Part model, mm, in its own coordinate system. A direction names the side the tool comes from. Round coordinates to 2 decimals unless told otherwise and drop trailing zeros. Loops run counter-clockwise (first coordinate to the right, second up) from the corner with the lowest first, then second, coordinate; pieces in that order, holes last. Notation, with made-up numbers: M 36,77.5 L 55,77.5 A15 ccw 55,84.5 Z; hole C 25.5,20.25 d1. An arc over 180 degrees is marked long. Put each result on its own line as item: value. Start each with the question number.
```python
from build123d import *

# Parameters (mm, degrees)
BOSS_EXTRUDE2_START  = 12.7
BOSS_EXTRUDE2_DEPTH  = 12.7
BOSS_EXTRUDE3_DEPTH  = 12.7
SKETCH8_R            = 0.9525
CUT_EXTRUDE1_DEPTH   = 157.544227843
SKETCH9_R            = 0.9525
CUT_EXTRUDE2_DEPTH   = 164.292861742
SKETCH12_R           = 2.5527
BOSS_EXTRUDE10_DEPTH = 3.175


with BuildPart() as part:
    # Sweep1: sweep along a path in Sketch4
    with BuildLine(Plane.XY) as sweep1_path:
        Line((0, 0), (0, -92.964))
        ThreePointArc((0, -92.964), (0.223184633, -93.502815367), (0.762, -93.726))
        Line((0.762, -93.726), (93.726, -93.726))
    # Sketch3 → Sweep1 (sweep)
    with BuildSketch(Plane(origin=(0, 0, 0), x_dir=(1, 0, 0), z_dir=(0, 1, 0))):
        with BuildLine():
            Line((0, 16.62500014), (-25.4, 16.62500014))
            Line((-25.4, 16.62500014), (-25.4, 10.27500014))
            Line((-25.4, 10.27500014), (-6.985, 10.27500014))
            ThreePointArc((-6.985, 10.27500014), (-6.535987194, 10.089012946), (-6.35, 9.64000014))
            Line((-6.35, 9.64000014), (-6.35, -14.48999986))
            ThreePointArc((-6.35, -14.48999986), (-6.535987194, -14.939012666), (-6.985, -15.12499986))
            Line((-6.985, -15.12499986), (-25.4, -15.12499986))
            Line((-25.4, -15.12499986), (-25.4, -21.47499986))
            Line((-25.4, -21.47499986), (0, -21.47499986))
            Line((0, -21.47499986), (0, 16.62500014))
        make_face()
    sweep(path=sweep1_path.line)

    # Sketch6 → Boss-Extrude2 (add)
    with BuildSketch(Plane(origin=(93.726, 0, 0), x_dir=(0, 0, -1), z_dir=(1, 0, 0)).offset(BOSS_EXTRUDE2_START)):
        with BuildLine():
            Line((-18.04599986, -97.155), (13.19600014, -97.155))
            Line((13.19600014, -97.155), (13.19600014, -119.126))
            Line((13.19600014, -119.126), (10.27500014, -119.126))
            Line((10.27500014, -119.126), (10.27500014, -100.711))
            ThreePointArc((10.27500014, -100.711), (10.089012946, -100.261987194), (9.64000014, -100.076))
            Line((9.64000014, -100.076), (-14.48999986, -100.076))
            ThreePointArc((-14.48999986, -100.076), (-14.939012666, -100.261987194), (-15.12499986, -100.711))
            Line((-15.12499986, -100.711), (-15.12499986, -119.126))
            Line((-15.12499986, -119.126), (-18.04599986, -119.126))
            Line((-18.04599986, -119.126), (-18.04599986, -97.155))
        make_face()
    extrude(amount=-BOSS_EXTRUDE2_DEPTH)

    # Sketch7 → Boss-Extrude3 (add)
    with BuildSketch(Plane(origin=(0, 0, 0), x_dir=(1, 0, 0), z_dir=(0, 1, 0))):
        Polygon((-25.4, 13.45000014), (-25.4, 16.62500014), (0, 16.62500014), (0, -21.47499986), (-25.4, -21.47499986), (-25.4, -18.29999986), (-3.175, -18.29999986), (-3.175, 13.45000014), align=None)
    extrude(amount=BOSS_EXTRUDE3_DEPTH)

    # Sketch8 → Cut-Extrude1 (cut, through all)
    with BuildSketch(Plane.XZ.offset(100.076)):
        with Locations(Location((100.076, 8.13999986, 0), (0, 0, 270))):
            Circle(SKETCH8_R)
        with Locations(Location((100.076, -3.29000014, 0), (0, 0, 270))):
            Circle(SKETCH8_R)
    extrude(amount=-CUT_EXTRUDE1_DEPTH, mode=Mode.SUBTRACT)

    # Sketch9 → Cut-Extrude2 (cut, through all)
    with BuildSketch(Plane.ZY.offset(3.175)):
        with Locations((-3.29000014, 6.35)):
            Circle(SKETCH9_R)
        with Locations((8.13999986, 6.35)):
            Circle(SKETCH9_R)
    extrude(amount=-CUT_EXTRUDE2_DEPTH, mode=Mode.SUBTRACT)

    # Sketch12 → Boss-Extrude10 (add, symmetric)
    with BuildSketch(Plane.XY.offset(7.62)):
        with BuildLine():
            Line((0.762, -93.726), (25.622204075, -93.726))
            ThreePointArc((25.622204075, -93.726), (18.183696875, -75.542303125), (0, -68.103795925))
            Line((0, -68.103795925), (0, -92.964))
            ThreePointArc((0, -92.964), (0.223184633, -93.502815367), (0.762, -93.726))
        make_face()
        with Locations((11.43, -82.296)):
            Circle(SKETCH12_R, mode=Mode.SUBTRACT)
    extrude(amount=BOSS_EXTRUDE10_DEPTH, both=True)

    # Sketch14 → CSK for _6 Flat Head Machine Screw _100 (revolve, cut)
    with BuildSketch(Plane(origin=(100.076, -100.076, -3.29000014), x_dir=(0, 0, -1), z_dir=(1, 0, 0))):
        Polygon((0, 0), (0, 2.410824014), (1.89865, 1.27), (1.89865, 1.380025208), (3.5433, 0), align=None)
    revolve(axis=Axis((100.076, -106.426, -3.29000014), (0, 1, 0)), mode=Mode.SUBTRACT)

    # Sketch16 → CSK for _6 Flat Head Machine Screw _ 2 (revolve, cut)
    with BuildSketch(Plane(origin=(100.076, -100.076, 8.13999986), x_dir=(0, 0, -1), z_dir=(1, 0, 0))):
        Polygon((0, 0), (0, 2.410824014), (1.89865, 1.27), (1.89865, 1.380025208), (3.5433, 0), align=None)
    revolve(axis=Axis((100.076, -106.426, 8.13999986), (0, 1, 0)), mode=Mode.SUBTRACT)


solid = part.part
```
1. Cut at A-A, the plane y = -49. Give the cut face in (x, z) (3 decimals), and give its area (3 significant figures).
2. Mould opens along X. For faces 1 (the flat face through (93.726, -97, 1)), 2 (the flat face through (-14, 6, 18.3)), 3 (the cylindrical face through (-17.9, -111.3, -13.4)), 4 (the cylindrical face through (11.098, -79.765, 7.576)) say: released by +X, released by -X, zero draft, split by the parting line, or undercut.
3. Which spindle directions (+Z, -Z, +X, -X, +Y, -Y) get a long thin tool onto all of the face, cutting with end or side? Do faces 5 (the flat face through (-14, 6, -13.45)), 6 (the flat face through (100, -108, -13.196)), 7 (the flat face through (10, -86, 10.795)). Say none if no direction does.
4. Cut at B-B, the plane x = 60. Give the cut face in (y, z) (3 decimals).
5. Cut at C-C, the plane x = 11.43. Give the cut face in (y, z) (3 decimals), and give its area (3 significant figures).
6. Wall check: L1, parallel to Z at x = 57.5, y = -108 (3 decimals); L2, parallel to Z at x = 96.5, y = -105 (3 decimals); L3, parallel to X at y = -97.55, z = -3.29. Give the ranges that are in metal, low to high.
7. Drop flat-ended pins along their axis: pin 1 (4 mm diameter, centred on y = -53, z = 12.5, fed in from +X); pin 2 (10 mm diameter, centred on x = 100.5, z = 5.5, fed in from +Y) (3 decimals); pin 3 (4 mm diameter, centred on y = -3, z = -0.5, fed in from -X). Give the stop position or say it passes through.
Results list:
1. outline: M -25.4,-16.625 L 0,-16.625 L 0,21.475 L -25.4,21.475 L -25.4,15.125 L -6.985,15.125 A0.635 cw -6.35,14.49 L -6.35,-9.64 A0.635 cw -6.985,-10.275 L -25.4,-10.275 Z
1. area: 484 mm^2
2. face 1: released by +X
2. face 2: zero draft
2. face 3: released by -X
2. face 4: undercut
3. face 5: -X, +Y
3. face 6: -Z, +X, +Y, -Y
3. face 7: +Z, +X, +Y
4. outline: M -119.126,-16.625 L -93.726,-16.625 L -93.726,21.475 L -119.126,21.475 L -119.126,15.125 L -100.711,15.125 A0.635 cw -100.076,14.49 L -100.076,-9.64 A0.635 cw -100.711,-10.275 L -119.126,-10.275 Z
5. outline: M -119.126,-16.625 L -93.726,-16.625 L -93.726,4.445 L -84.849,4.445 L -84.849,10.795 L -93.726,10.795 L -93.726,21.475 L -119.126,21.475 L -119.126,15.125 L -100.711,15.125 A0.635 cw -100.076,14.49 L -100.076,-9.64 A0.635 cw -100.711,-10.275 L -119.126,-10.275 Z; M -79.743,4.445 L -70.709,4.445 L -70.709,10.795 L -79.743,10.795 Z
5. area: 598 mm^2
6. L1: z = -16.625 to -10.275, 15.125 to 21.475
6. L2: z = -13.196 to -10.275, 15.125 to 18.046
6. L3: x = -4.67 to 99.12, 101.03 to 106.43
7. pin 1: stops at x = 0
7. pin 2: stops at y = -97.155
7. pin 3: stops at x = -6.35
